CAD build for the part. Positions are in the model's coordinates, mm. A direction names the side the tool comes from. Round coordinates to 2 decimals unless told otherwise and drop trailing zeros. Loops run counter-clockwise (first coordinate to the right, second up) from the corner with the lowest first, then second, coordinate; pieces in that order, holes last. Notation, with made-up numbers: (58.5, 21.25) - (114.5, 21.25) arc R23 cw to (114.5, 52.25) - close; hole circle Ø2 at (53, 0.25). An arc over 180 degrees is marked (long way). Use one line per item in the form item = value.
from build123d import *

# Parameters (mm, degrees)
SKETCH1_W           = 165.1
SKETCH1_H           = 88.9
BOSS_EXTRUDE1_DEPTH = 43.18
SKETCH2_W           = 50.8
SKETCH2_H           = 35.56
CUT_EXTRUDE1_DEPTH  = 40.64
CUT_EXTRUDE2_DEPTH  = 162.56
SKETCH4_W           = 2.54
SKETCH4_H           = 25.4
CUT_EXTRUDE3_DEPTH  = 6.35
FILLET1_START       = -1
FILLET1_DEPTH       = 45
FILLET2_R           = 1.27


with BuildPart() as part:
    # Sketch1 → Boss-Extrude1 (new body)
    with BuildSketch(Plane(origin=(0, 0, 0), x_dir=(1, 0, 0), z_dir=(0, 1, 0))):
        with Locations((82.55, 44.45)):
            Rectangle(SKETCH1_W, SKETCH1_H)
    extrude(amount=BOSS_EXTRUDE1_DEPTH)

    # Sketch2 → Cut-Extrude1 (cut)
    with BuildSketch(Plane(origin=(0, 43.18, 0), x_dir=(1, 0, 0), z_dir=(0, 1, 0))):
        with Locations((29.21, 63.5)):
            Rectangle(SKETCH2_W, SKETCH2_H)
        with Locations((29.21, 25.4)):
            Rectangle(SKETCH2_W, SKETCH2_H)
        with Locations((82.55, 63.5)):
            Rectangle(SKETCH2_W, SKETCH2_H)
        with Locations((135.89, 63.5)):
            Rectangle(SKETCH2_W, SKETCH2_H)
        with Locations((135.89, 25.4)):
            Rectangle(SKETCH2_W, SKETCH2_H)
        with Locations((82.55, 25.4)):
            Rectangle(SKETCH2_W, SKETCH2_H)
    extrude(amount=-CUT_EXTRUDE1_DEPTH, mode=Mode.SUBTRACT)

    # Sketch3 → Cut-Extrude2 (cut)
    with BuildSketch(Plane(origin=(165.1, 0, 0), x_dir=(0, 0, -1), z_dir=(1, 0, 0))):
        Polygon((2.54, 40.64), (7.62, 40.64), (7.62, 43.18), (81.28, 43.18), (81.28, 40.64), (86.36, 40.64), (86.36, 36.83), (2.54, 36.83), align=None)
    extrude(amount=-CUT_EXTRUDE2_DEPTH, mode=Mode.SUBTRACT)

    # Sketch4 → Cut-Extrude3 (cut)
    with BuildSketch(Plane(origin=(0, 43.18, 0), x_dir=(1, 0, 0), z_dir=(0, 1, 0))):
        with Locations((1.27, 44.45)):
            Rectangle(SKETCH4_W, SKETCH4_H)
    extrude(amount=-CUT_EXTRUDE3_DEPTH, mode=Mode.SUBTRACT)

    # Fillet1: read off the stored shape, not the designer's step
    # Fillet1 outline → Fillet1 (cut)
    with BuildSketch(Plane(origin=(0, 0, 0), x_dir=(1, 0, 0), z_dir=(0, 1, 0)).offset(FILLET1_START)):
        with BuildLine():
            Line((0, 88.9), (0, 86.36))
            ThreePointArc((0, 86.36), (0.743948776, 88.156051224), (2.54, 88.9))
            Line((2.54, 88.9), (0, 88.9))
        make_face()
        with BuildLine():
            ThreePointArc((2.54, 0), (0.743948776, 0.743948776), (0, 2.54))
            Line((0, 2.54), (0, 0))
            Line((0, 0), (2.54, 0))
        make_face()
        with BuildLine():
            Line((165.1, 88.9), (162.56, 88.9))
            ThreePointArc((162.56, 88.9), (164.356051224, 88.156051224), (165.1, 86.36))
            Line((165.1, 86.36), (165.1, 88.9))
        make_face()
        with BuildLine():
            ThreePointArc((165.1, 2.54), (164.356051224, 0.743948776), (162.56, 0))
            Line((162.56, 0), (165.1, 0))
            Line((165.1, 0), (165.1, 2.54))
        make_face()
    extrude(amount=FILLET1_DEPTH, mode=Mode.SUBTRACT)

    # Fillet2
    fillet2_edges = [part.edges().sort_by_distance(p)[0] for p in [
        (1.27, 36.83, -57.15),
        (1.27, 36.83, -31.75),
        (1.27, 43.18, -31.75),
        (1.27, 43.18, -57.15),
        (57.15, 19.685, -7.62),
        (57.15, 19.685, -43.18),
        (107.95, 19.685, -43.18),
        (107.95, 19.685, -7.62),
        (110.49, 19.685, -45.72),
        (110.49, 19.685, -81.28),
        (161.29, 19.685, -81.28),
        (161.29, 19.685, -45.72),
        (57.15, 19.685, -45.72),
        (57.15, 19.685, -81.28),
        (107.95, 19.685, -81.28),
        (107.95, 19.685, -45.72),
        (3.81, 19.685, -7.62),
        (3.81, 19.685, -43.18),
        (54.61, 19.685, -43.18),
        (54.61, 19.685, -7.62),
        (110.49, 19.685, -7.62),
        (110.49, 19.685, -43.18),
        (161.29, 19.685, -43.18),
        (161.29, 19.685, -7.62),
        (3.81, 19.685, -45.72),
        (3.81, 19.685, -81.28),
        (54.61, 19.685, -81.28),
        (54.61, 19.685, -45.72),
    ]]
    fillet(fillet2_edges, radius=FILLET2_R)


solid = part.part
1) Two-plate mould, pull along X, no slides. Class faces 1 (the flat face through (85, 39, -86.36)), 2 (the flat face through (0, 21, -44)), 3 (the flat face through (29, 20, -43.18)): +X half, -X half, draft (parallel to the pull), parting line (faces both ways), or undercut.
Report:
face_1 = draft
face_2 = -X half
face_3 = undercut
2) Slice it at C-C (y = 17). State how many separate pieces and enclosed holes the cut face has, plus the area to 3 significant figures.
Report:
separate_pieces = 1
enclosed_holes = 6
area = 3,840 mm^2
3) Tool access for faces 4 (the flat face through (3.81, 20, -25)), 5 (the flat face through (81, 21, 0)), 6 (the flat face through (85, 40.64, -5)): list every direction of +Z, -Z, +X, -X, +Y, -Y with a clear straight run to the whole face (end or side of a thin tool).
Report:
face_4 = +Y
face_5 = +Z, +X, -X, +Y, -Y
face_6 = +X
4) Slice it at A-A (z = -49). Write the cut outline in (x, y), plus the area to 3 significant figures.
Report:
outline = (0, 0) - (165.1, 0) - (165.1, 36.83) - (161.29, 36.83) - (161.29, 2.54) - (110.49, 2.54) - (110.49, 36.83) - (107.95, 36.83) - (107.95, 2.54) - (57.15, 2.54) - (57.15, 36.83) - (54.61, 36.83) - (54.61, 2.54) - (3.81, 2.54) - (3.81, 36.83) - (0, 36.83) - close
area = 855 mm^2
5) Slice it at B-B (x = 83.5). Write the cut outline in (y, z), plus the area to 3 significant figures.
Report:
outline = (0, -88.9) - (43.18, -88.9) - (43.18, -81.28) - (40.64, -81.28) - (40.64, -86.36) - (36.83, -86.36) - (36.83, -81.28) - (2.54, -81.28) - (2.54, -45.72) - (36.83, -45.72) - (36.83, -43.18) - (2.54, -43.18) - (2.54, -7.62) - (36.83, -7.62) - (36.83, -2.54) - (40.64, -2.54) - (40.64, -7.62) - (43.18, -7.62) - (43.18, 0) - (0, 0) - close
area = 894 mm^2
6) Slice it at D-D (z = -11). Write the cut outline in (x, y), plus the area to 3 significant figures.
Report:
outline = (0, 0) - (165.1, 0) - (165.1, 36.83) - (161.29, 36.83) - (161.29, 2.54) - (110.49, 2.54) - (110.49, 36.83) - (107.95, 36.83) - (107.95, 2.54) - (57.15, 2.54) - (57.15, 36.83) - (54.61, 36.83) - (54.61, 2.54) - (3.81, 2.54) - (3.81, 36.83) - (2.54, 36.83) - (2.54, 43.18) - (0, 43.18) - close
area = 871 mm^2
7) Flat gauge pins, fed straight in: pin 1 (12 mm diameter, centred on x = 17.5, z = -27.5, fed in from +Y); pin 2 (8 mm diameter, centred on x = 97, z = -15, fed in from -Y); pin 3 (1.3 mm diameter, centred on x = 1, y = 41, fed in from -Z). Where does each tip first touch, or does it go through?
Report:
pin_1 = 2.54
pin_2 = 0
pin_3 = -88.74
8) Drill centre lines: probe 1 along Z at (x, y) = (122, 10.5); probe 2 along X at (y, z) = (26.5, -28); probe 3 along Y at (x, z) = (60.5, -83.5). Where is each one in solid material? Low to high.
Report:
probe_1 = -88.9 to -81.28, -45.72 to -43.18, -7.62 to 0
probe_2 = 0 to 3.81, 54.61 to 57.15, 107.95 to 110.49, 161.29 to 165.1
probe_3 = 0 to 36.83, 40.64 to 43.18
